Print and shaded views of the part. All mm, measured from the part's lowest x, y and z. Coordinates: 2 decimals unless noted, no trailing zeros. Loops run counter-clockwise (first coordinate to the right, second up) from the corner with the lowest first, then second, coordinate; pieces in that order, holes last. Notation, with made-up numbers: M 1,70 L 43,70 A29 cw 43,90 Z; hole C -27.5,3 d4. An arc over 180 degrees is marked long. Answer as a JSON object with one key per item and string values. Group by question number.
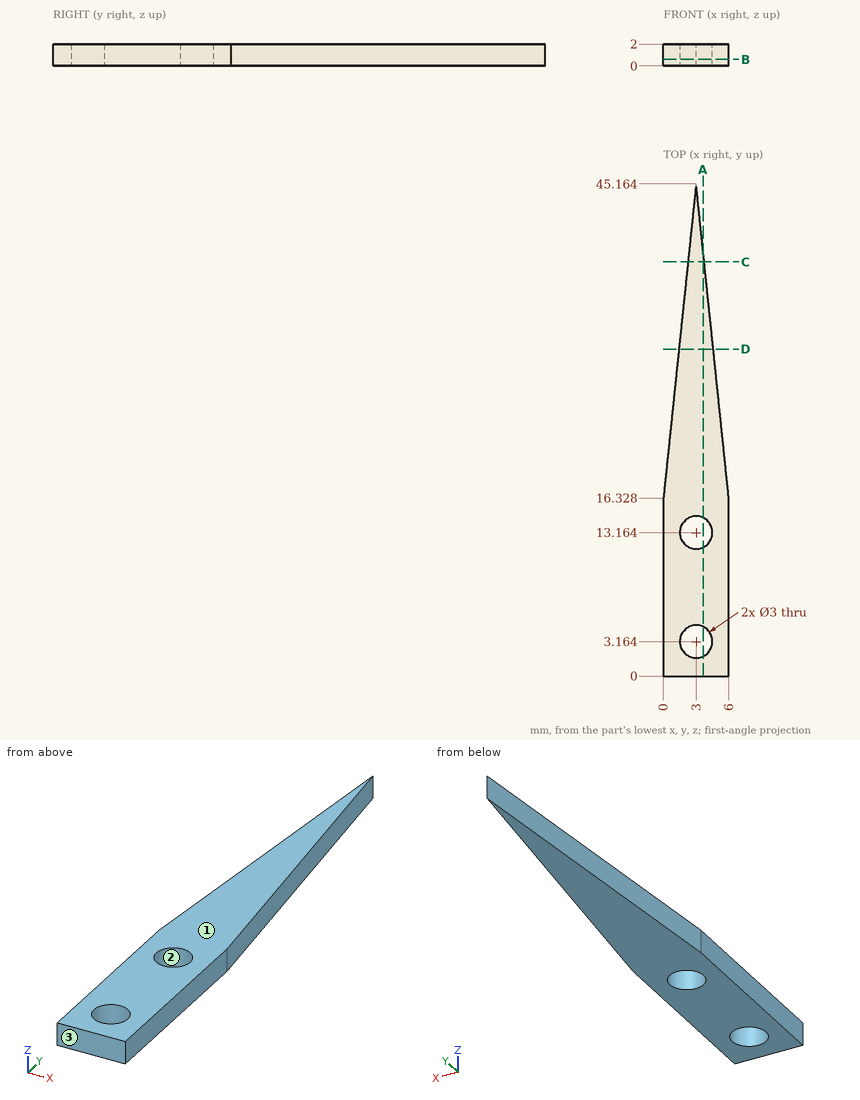
Item 1: Slice it at B-B, the plane z = 0.6. Write the cut outline in (x, y).
Item 2: Drill centre lines: L1, parallel to X at y = 22.5, z = 1.05; L2, parallel to X at y = 32, z = 1.6; L3, parallel to X at y = 4, z = 1.9 (1 decimal). Where is each one in solid material? Low to high. Write a range as from..to.
Item 3: Slice it at D-D, the plane y = 30. Write the cut outline in (x, z).
Item 4: Slice it at A-A, the plane x = 3.65. Write the cut outline in (y, z).
Item 5: Slice it at C-C, the plane y = 38. Write the cut outline in (x, z) (1 decimal).
Item 6: Pull direction Y, two halves, no side cores. Call the marked faces 1, 2 and 3: released by +Y, released by -Y, zero draft, split by the parting line, or undercut.
Computed:
{
 "1": {"outline": "M 0,0 L 6,0 L 6,16.33 L 3,45.16 L 0,16.33 Z; hole C 3,3.16 d3; hole C 3,13.16 d3"},
 "2": {"L1": "0.64..5.36", "L2": "1.63..4.37", "L3": "0..1.8, 4.2..6"},
 "3": {"outline": "M 1.42,0 L 4.58,0 L 4.58,2 L 1.42,2 Z"},
 "4": {"outline": "M 0,0 L 1.81,0 L 1.81,2 L 0,2 Z; M 4.52,0 L 11.81,0 L 11.81,2 L 4.52,2 Z; M 14.52,0 L 38.92,0 L 38.92,2 L 14.52,2 Z"},
 "5": {"outline": "M 2.3,0 L 3.7,0 L 3.7,2 L 2.3,2 Z"},
 "6": {"face 1": "zero draft", "face 2": "undercut", "face 3": "released by -Y"}
}
